Geometry check sheet. Reference: the model listing, model coordinates, mm. Round coordinates to 2 decimals unless told otherwise and drop trailing zeros. Loops run counter-clockwise (first coordinate to the right, second up) from the corner with the lowest first, then second, coordinate; pieces in that order, holes last. Notation, with made-up numbers: (27, -4) -> (34, -4) arc R15 ccw to (34, 21) -> close; hole circle Ø4 at (33, 67.5). An arc over 180 degrees is marked (long way). Use one line per item in the form item = value.
from build123d import *

# Parameters (mm, degrees)
F0_R     = 1.096214
F0_R_2   = 5.824912
F0_R_3   = 1.180333
F0_R_4   = 1.117938
F0_R_5   = 5.484301
F1_DEPTH = 12.7


with BuildPart() as f1:
    # F0 (on Top) → F1 (new body)
    with BuildSketch(Plane.XY):
        Polygon((-7.145739, 28.330129), (-39.747888, 46.809014), (-39.152107, -28.138449), (-6.847849, -9.143603), align=None)
        with Locations((-37.967294, -22.222633)):
            Circle(F0_R, mode=Mode.SUBTRACT)
        with Locations((-19.233698, -1.718403)):
            Circle(F0_R_2, mode=Mode.SUBTRACT)
        with Locations((-9.175166, -7.444786)):
            Circle(F0_R_3, mode=Mode.SUBTRACT)
        with Locations((-37.937455, 43.433934)):
            Circle(F0_R_4, mode=Mode.SUBTRACT)
        with Locations((-20.150922, 20.580299)):
            Circle(F0_R_5, mode=Mode.SUBTRACT)
        with Locations((-9.675507, 27.038466)):
            Circle(F0_R_4, mode=Mode.SUBTRACT)
    extrude(amount=F1_DEPTH)


solid = f1.part
1. Section check C-C (z = 1). Record the boundary of the cut face in (x, y), then the cut area to 3 significant figures.
Return value:
outline = (-39.75, 46.81) -> (-39.15, -28.14) -> (-6.85, -9.14) -> (-7.15, 28.33) -> close; hole circle Ø2.19 at (-37.97, -22.22); hole circle Ø2.24 at (-37.94, 43.43); hole circle Ø10.97 at (-20.15, 20.58); hole circle Ø11.65 at (-19.23, -1.72); hole circle Ø2.24 at (-9.68, 27.04); hole circle Ø2.36 at (-9.18, -7.44)
area = 1,610 mm2
2. Mould release check, pull along Y, two halves, no side actions. Record for faces 1 (the flat face through (-27, 10, 0)), 2 (the flat face through (-23.226, -18.774, 6.261)), 3 (the cylindrical face through (-38.775, -21.482, 6.261)): released by +Y, released by -Y, zero draft, split by the parting line, or undercut.
Return value:
face_1 = zero draft
face_2 = released by -Y
face_3 = undercut
3. Section check A-A (x = -20.5). Record the boundary of the cut face in (y, z).
Return value:
outline = (-17.17, 0) -> (-7.4, 0) -> (-7.4, 12.7) -> (-17.17, 12.7) -> close; (3.97, 0) -> (15.11, 0) -> (15.11, 12.7) -> (3.97, 12.7) -> close; (26.05, 0) -> (35.9, 0) -> (35.9, 12.7) -> (26.05, 12.7) -> close
4. Section check B-B (y = 22). Record the boundary of the cut face in (x, z).
Return value:
outline = (-39.55, 0) -> (-25.45, 0) -> (-25.45, 12.7) -> (-39.55, 12.7) -> close; (-14.85, 0) -> (-7.1, 0) -> (-7.1, 12.7) -> (-14.85, 12.7) -> close
5. Material ranges on line 1 along Y through (x, z) = (-20, 10.25); line 2 along Y through (x, z) = (-37.5, 10.75); line 3 along X through (y, z) = (1, 2.5), recorded low to high.
Return value:
line_1 = -16.88 to -7.49, 4.06 to 15.1, 26.06 to 35.62
line_2 = -27.17 to -23.21, -21.23 to 42.41, 44.46 to 45.53
line_3 = -39.38 to -24.39, -14.08 to -6.93
6. Gauge pin test, flat ends, axial feed: pin 1 (2 mm diameter, centred on y = 7.5, z = 9.5, fed in from -X); pin 2 (1 mm diameter, centred on x = -35, z = 6, fed in from +Y); pin 3 (1.5 mm diameter, centred on x = -16.5, z = 3.5, fed in from +Y). Record the tip position at first contact, or that the pin passes through.
Return value:
pin_1 = -39.44
pin_2 = 44.4
pin_3 = 34.06
7. Section check D-D (x = -16). Record the boundary of the cut face in (y, z).
Return value:
outline = (-14.53, 0) -> (-6.56, 0) -> (-6.56, 12.7) -> (-14.53, 12.7) -> close; (3.13, 0) -> (17, 0) -> (17, 12.7) -> (3.13, 12.7) -> close; (24.16, 0) -> (33.35, 0) -> (33.35, 12.7) -> (24.16, 12.7) -> close
